Geometry check sheet. Reference: the model listing, model coordinates, mm. A direction names the side the tool comes from. Give positions to 0.01 mm unless a question says otherwise; leave off trailing zeros. Loops run counter-clockwise (first coordinate to the right, second up) from the corner with the lowest first, then second, coordinate; pieces in that order, holes last. Notation, with made-up numbers: (41, 67.25) - (72, 67.25) arc R19 cw to (72, 71.25) - close; hole circle Ø6 at (-10, 47). An arc over 180 degrees is marked (long way). Use a Markdown table: item, result. Add a question column.
1. Set-up check for faces 5 (the flat face through (28.33, -2.99, 1.48)), 6 (the flat face through (-1, 21.175, 1)), 7 (the flat face through (-57.166, -3.051, 1.479)): record each of +Z, -Z, +X, -X, +Y, -Y from which the full face is reachable in a straight line by a thin tool's end or side.
2. Cross-section at A-A on y = 12.5. Enter the section's corners in (x, z), and give its area (3 significant figures).
3. Cross-section at D-D on x = 22.5. Enter the section's corners in (y, z), and give its area (3 significant figures).
4. Cross-section at B-B on z = 1.85. Count the separate pieces of the cut face and the enclosed holes in it, and give its area (3 significant figures).
5. Material ranges on L1, parallel to X at y = 10, z = 1.95; L2, parallel to X at y = -13, z = 1.35; L3, parallel to Y at x = -56, z = 1.45, recorded low to high.
6. Depth check by flat-ended pin: P1, Ø0.6, axis at x = 26, z = 2, coming from the -Y side; P2, Ø0.6, axis at x = -54.5, z = 1.5, coming from the +Y side. Enter the tip coordinate at first touch or a pass-through.
7. Cross-section at C-C on y = -46.5. Enter the section's corners in (x, z).
8. Draft check along X on faces 1 (the flat face through (25.483, 52.85, 1.479)), 2 (the flat face through (-59.447, -80, 1)), 3 (the flat face through (-29.447, -67, 1)), 4 (the flat face through (-2.447, 11, 1)). Enter one of: pulls with the +X half, pulls with the -X half, needs draft (parallel to the pull), parting line crosses it, or undercut.
from build123d import *

# Parameters (mm, degrees)
SKETCH1_R           = 1.65
SKETCH1_W           = 3
SKETCH1_H           = 20
BOSS_EXTRUDE2_DEPTH = 3


with BuildPart() as part:
    # Sketch1 → Boss-Extrude2 (new body)
    with BuildSketch(Plane.XY):
        Polygon((-59.447183423, 47.780041818), (-49.447183423, 57.780041818), (20.552816577, 57.780041818), (30.552816577, 47.780041818), (30.552816577, -0.7691812), (26.052816577, -5.2691812), (25.552816577, -5.2691812), (25.552816577, -50.590735163), (26.052816577, -50.590735163), (30.552816577, -55.090735163), (30.552816577, -103.639958182), (20.552816577, -113.639958182), (-49.447183423, -113.639958182), (-59.447183423, -103.639958182), (-59.447183423, -55.090735163), (-54.947183423, -50.590735163), (-54.447183423, -50.590735163), (-54.447183423, -5.2691812), (-54.947183423, -5.2691812), (-59.447183423, -0.7691812), align=None)
        with Locations((-39.447183423, 52.780041818)):
            Circle(SKETCH1_R, mode=Mode.SUBTRACT)
        with Locations((10.552816577, 52.780041818)):
            Circle(SKETCH1_R, mode=Mode.SUBTRACT)
        with Locations(Location((10.552816577, -108.639958182, 0), (0, 0, 180))):
            Circle(SKETCH1_R, mode=Mode.SUBTRACT)
        with Locations(Location((-39.447183423, -108.639958182, 0), (0, 0, 180))):
            Circle(SKETCH1_R, mode=Mode.SUBTRACT)
        with Locations((-27.947183423, 11.175041818)):
            Rectangle(SKETCH1_W, SKETCH1_H, mode=Mode.SUBTRACT)
        with Locations((-0.947183423, 11.175041818)):
            Rectangle(SKETCH1_W, SKETCH1_H, mode=Mode.SUBTRACT)
        with Locations((-0.947183423, -67.034958182)):
            Rectangle(SKETCH1_W, SKETCH1_H, mode=Mode.SUBTRACT)
        with Locations((-27.947183423, -67.034958182)):
            Rectangle(SKETCH1_W, SKETCH1_H, mode=Mode.SUBTRACT)
    extrude(amount=BOSS_EXTRUDE2_DEPTH)


solid = part.part
Values found:
| question | item | result |
|---|---|---|
| 1 | face 5 | +Z, -Z, +X |
| 1 | face 6 | +Z, -Z |
| 1 | face 7 | +Z, -Z, -X |
| 2 | outline | (-59.45, 0) - (-29.45, 0) - (-29.45, 3) - (-59.45, 3) - close; (-26.45, 0) - (-2.45, 0) - (-2.45, 3) - (-26.45, 3) - close; (0.55, 0) - (30.55, 0) - (30.55, 3) - (0.55, 3) - close |
| 2 | area | 252 mm2 |
| 3 | outline | (-111.69, 0) - (55.83, 0) - (55.83, 3) - (-111.69, 3) - close |
| 3 | area | 503 mm2 |
| 4 | separate pieces | 1 |
| 4 | enclosed holes | 8 |
| 4 | area | 14,500 mm2 |
| 5 | L1 | x = -59.45 to -29.45, -26.45 to -2.45, 0.55 to 30.55 |
| 5 | L2 | x = -54.45 to 25.55 |
| 5 | L3 | y = -107.09 to -51.64, -4.22 to 51.23 |
| 6 | P1 | stops at y = -108.49 |
| 6 | P2 | stops at y = 53.03 |
| 7 | outline | (-54.45, 0) - (25.55, 0) - (25.55, 3) - (-54.45, 3) - close |
| 8 | face 1 | pulls with the +X half |
| 8 | face 2 | pulls with the -X half |
| 8 | face 3 | undercut |
| 8 | face 4 | undercut |
